Work out the finished part from the listing and answer in its coordinate system (mm). Give positions to 0.01 mm unless a question says otherwise; leave off trailing zeros. Loops run counter-clockwise (first coordinate to the right, second up) from the corner with the lowest first, then second, coordinate; pieces in that order, holes last. Notation, with made-up numbers: M 81.25,12.5 L 94.25,12.5 A19 ccw 94.25,26.5 Z; hole C 56.5,44.5 d9. An arc over 180 degrees is marked long. Answer as a JSON object with one key per item and string values. Group by question number.
```python
from build123d import *

# Parameters (mm, degrees)
F0_W     = 20
F0_H     = 21.1
F1_DEPTH = 15.25
F4_DEPTH = 20.001
F5_R     = 0.6


with BuildPart() as f1:
    # F0 (on Top) → F1 (new body)
    with BuildSketch(Plane.XY):
        with Locations((10, 10.55)):
            Rectangle(F0_W, F0_H)
    extrude(amount=F1_DEPTH)

    # F3 (on face) → F4 (cut, through all)
    with BuildSketch(Plane.YZ.offset(20)):
        with BuildLine():
            Line((3.9, 15.25), (1.25, 15.25))
            Line((1.25, 15.25), (1.575, 3.2229775179))
            ThreePointArc((1.575, 3.2229775179), (2.575, 2.2496349594), (3.575, 3.2229775179))
            Line((3.575, 3.2229775179), (3.9, 15.25))
        make_face()
        with BuildLine():
            Line((7.9, 15.25), (5.25, 15.25))
            Line((5.25, 15.25), (5.575, 3.2229775179))
            ThreePointArc((5.575, 3.2229775179), (6.575, 2.2496349594), (7.575, 3.2229775179))
            Line((7.575, 3.2229775179), (7.9, 15.25))
        make_face()
        with BuildLine():
            Line((11.9, 15.25), (9.25, 15.25))
            Line((9.25, 15.25), (9.575, 3.2229775179))
            ThreePointArc((9.575, 3.2229775179), (10.575, 2.2496349594), (11.575, 3.2229775179))
            Line((11.575, 3.2229775179), (11.9, 15.25))
        make_face()
        with BuildLine():
            Line((15.9, 15.25), (13.25, 15.25))
            Line((13.25, 15.25), (13.575, 3.2229775179))
            ThreePointArc((13.575, 3.2229775179), (14.575, 2.2496349594), (15.575, 3.2229775179))
            Line((15.575, 3.2229775179), (15.9, 15.25))
        make_face()
        with BuildLine():
            Line((19.575, 3.2229775179), (19.9, 15.25))
            Line((19.9, 15.25), (17.25, 15.25))
            Line((17.25, 15.25), (17.575, 3.2229775179))
            ThreePointArc((17.575, 3.2229775179), (18.575, 2.2496349594), (19.575, 3.2229775179))
        make_face()
    extrude(amount=-F4_DEPTH, mode=Mode.SUBTRACT)

    # F5
    f5_edges = [f1.edges().sort_by_distance(p)[0] for p in [
        (10, 0, 15.25),
        (10, 1.25, 15.25),
        (10, 3.9, 15.25),
        (10, 5.25, 15.25),
        (10, 7.9, 15.25),
        (10, 9.25, 15.25),
        (10, 11.9, 15.25),
        (10, 13.25, 15.25),
        (10, 15.9, 15.25),
        (10, 17.25, 15.25),
        (10, 19.9, 15.25),
        (10, 21.1, 15.25),
    ]]
    fillet(f5_edges, radius=F5_R)


solid = f1.part
```
Item 1: A cutting plane is placed at C-C (y = 19). Determine the outline of the cut face in (x, z).
Item 2: A cutting plane is placed at A-A (z = 4.75). Determine the outline of the cut face in (x, y), and give its area (3 significant figures).
Item 3: Find the intervals of material crossed by probe 1 along Y at (x, z) = (9.5, 5.5); probe 2 along Y at (x, z) = (14.25, 9.5); probe 3 along Z at (x, y) = (2.25, 4), in increasing order. Write a range as [from, to].
Item 4: A cutting plane is placed at B-B (z = 9.75). Determine the outline of the cut face in (x, y), and give its area (3 significant figures).
Item 5: Given pin 1 Ø1 at (x, y) = (3.5, 5.5) entering from +Z, flat-ended and moving along its own axis, determine where the tip first touches the part or whether it passes through.
Item 6: For a pull along Y with two mould halves and no side action, classify faces 1 (the flat face through (10, 0, 7)), 2 (the cylindrical face through (10.14, 14.55, 2.25)), 3 (the flat face through (10, 11, 0)) as pulls with the +Y half, pulls with the -Y half, needs draft (parallel to the pull), parting line crosses it, or undercut.
Item 7: A cutting plane is placed at D-D (y = 2.25). Determine the outline of the cut face in (x, z).
The answers:
{
 "1": {"outline": "M 0,0 L 20,0 L 20,2.34 L 0,2.34 Z"},
 "2": {"outline": "M 0,0 L 20,0 L 20,1.53 L 0,1.53 Z; M 0,3.62 L 20,3.62 L 20,5.53 L 0,5.53 Z; M 0,7.62 L 20,7.62 L 20,9.53 L 0,9.53 Z; M 0,11.62 L 20,11.62 L 20,13.53 L 0,13.53 Z; M 0,15.62 L 20,15.62 L 20,17.53 L 0,17.53 Z; M 0,19.62 L 20,19.62 L 20,21.1 L 0,21.1 Z", "area": "214 mm^2"},
 "3": {"probe 1": "y = [0, 1.51], [3.64, 5.51], [7.64, 9.51], [11.64, 13.51], [15.64, 17.51], [19.64, 21.1]", "probe 2": "y = [0, 1.41], [3.74, 5.41], [7.74, 9.41], [11.74, 13.41], [15.74, 17.41], [19.74, 21.1]", "probe 3": "z = [0, 15]"},
 "4": {"outline": "M 0,0 L 20,0 L 20,1.4 L 0,1.4 Z; M 0,3.75 L 20,3.75 L 20,5.4 L 0,5.4 Z; M 0,7.75 L 20,7.75 L 20,9.4 L 0,9.4 Z; M 0,11.75 L 20,11.75 L 20,13.4 L 0,13.4 Z; M 0,15.75 L 20,15.75 L 20,17.4 L 0,17.4 Z; M 0,19.75 L 20,19.75 L 20,21.1 L 0,21.1 Z", "area": "187 mm^2"},
 "5": {"pin 1": "stops at z = 15.15"},
 "6": {"face 1": "pulls with the -Y half", "face 2": "undercut", "face 3": "needs draft"},
 "7": {"outline": "M 0,0 L 20,0 L 20,2.3 L 0,2.3 Z"}
}
